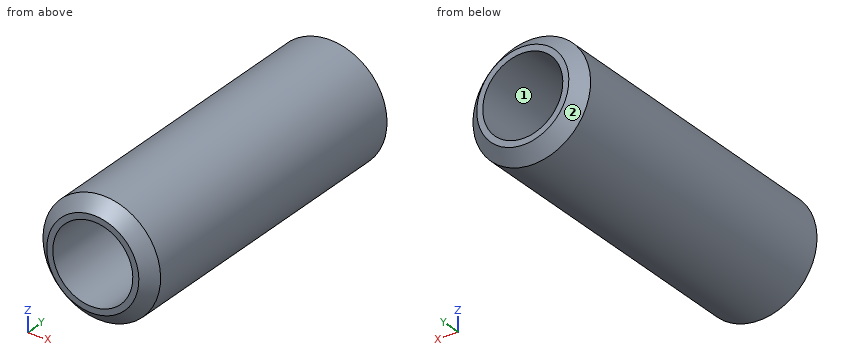
from build123d import *

# Parameters (mm, degrees)
SKETCH1_R           = 25
BOSS_EXTRUDE1_DEPTH = 147.222688
SKETCH2_R           = 17.014514558
CUT_EXTRUDE1_DEPTH  = 152.408453733
CHAMFER1_SIZE       = 5.419405


with BuildPart() as part:
    # Sketch1 → Boss-Extrude1 (new body)
    with BuildSketch(Plane(origin=(0, 0, 0), x_dir=(1, 0, 0), z_dir=(0, 1, 0))):
        with Locations(Location((0, 0, 0), (0, 0, 270))):
            Circle(SKETCH1_R)
    extrude(amount=BOSS_EXTRUDE1_DEPTH)

    # Sketch2 → Cut-Extrude1 (cut, through all)
    with BuildSketch(Plane(origin=(0, 0, 0), x_dir=(1, 0, 0), z_dir=(0, 1, 0))):
        with Locations(Location((0, 0, 0), (0, 0, 270))):
            Circle(SKETCH2_R)
    extrude(amount=CUT_EXTRUDE1_DEPTH, mode=Mode.SUBTRACT)

    # Chamfer1
    chamfer1_edges = [part.edges().sort_by_distance(p)[0] for p in [
        (0, 0, -25),
        (0, 147.222688, -25),
    ]]
    chamfer(chamfer1_edges, length=CHAMFER1_SIZE)


solid = part.part
Could you check a few things on this model? Use its own coordinates, in mm. Face numbers are marked on the shaded views. Round coordinates to 2 decimals unless told otherwise and drop trailing zeros. Write each loop counter-clockwise with the first axis right and the second up, starting at its lowest first coordinate (ties: lowest second). Pieces come first, ordered by that corner, then holes. Notation, with made-up numbers: (29.5, -27.5) - (82.5, -27.5) arc R21 ccw to (82.5, 5.5) - close; hole circle Ø6 at (6, -31). An arc over 180 degrees is marked (long way). Put each result on its own line as item: value. Start each with the question number.
(1) I want a section at A-A, the plane x = 0. Please give me the cut outline in (y, z).
(2) I need wall thicknesses on probe 1 along X at (y, z) = (74, 0); probe 2 along Z at (x, y) = (1, 42); probe 3 along Z at (x, y) = (6.5, 87). Which ranges of each line are inside material? Lowest first, please.
(3) Thinking about a two-plate mould opening in Z: for the marked faces 1 and 2, which applies, released by +Z, released by -Z, zero draft, split by the parting line, or undercut?
(4) I want a section at C-C, the plane y = 34.5. Please give me the cut outline in (x, z), plus the area to 3 significant figures.
(5) I want a section at B-B, the plane z = 0. Please give me the cut outline in (x, y), plus the area to 3 significant figures.
(6) Will these pins go through, and if not, where does the flat tip stop? pin 1 (3 mm diameter, centred on y = 89, z = -11, fed in from -X); pin 2 (1 mm diameter, centred on x = 17.5, z = 11.5, fed in from +Y); pin 3 (3 mm diameter, centred on x = 9.5, y = 124, fed in from +Z).
Here are the results:
1. outline: (0, -19.58) - (5.42, -25) - (141.8, -25) - (147.22, -19.58) - (147.22, -17.01) - (0, -17.01) - close; (0, 17.01) - (147.22, 17.01) - (147.22, 19.58) - (141.8, 25) - (5.42, 25) - (0, 19.58) - close
2. probe 1: x = -25 to -17.01, 17.01 to 25
2. probe 2: z = -24.98 to -16.99, 16.99 to 24.98
2. probe 3: z = -24.14 to -15.72, 15.72 to 24.14
3. face 1: undercut
3. face 2: split by the parting line
4. outline: circle Ø50 at (0, 0); hole circle Ø34.03 at (0, 0)
4. area: 1,050 mm^2
5. outline: (-25, 5.42) - (-19.58, 0) - (-17.01, 0) - (-17.01, 147.22) - (-19.58, 147.22) - (-25, 141.8) - close; (17.01, 0) - (19.58, 0) - (25, 5.42) - (25, 141.8) - (19.58, 147.22) - (17.01, 147.22) - close
5. area: 2,290 mm^2
6. pin 1: stops at x = -23.12
6. pin 2: stops at y = 146.36
6. pin 3: stops at z = 23.69
